from build123d import *

# Parameters (mm, degrees)
F0_W        = 85
F0_H        = 85
F1_DEPTH    = 3
F2_R        = 5
F3_DEPTH    = 7
F4_R        = 8
F5_R        = 2
F6_T1_DEPTH = 7


# Not quite as in the source:
# - a fillet or chamfer that OpenCascade refuses, or shapes differently, is made with other operations: its cross-section is extruded or revolved along the edge and cut away or added


with BuildPart() as f1:
    # F0 (on Top) → F1 (new body)
    with BuildSketch(Plane.XY):
        Rectangle(F0_W, F0_H)
        Polygon((-37.5, -6), (-37.5, 6), (-37.5, 37.5), (37.5, 37.5), (37.5, 6), (37.5, -6), (37.5, -37.5), (-37.5, -37.5), align=None, mode=Mode.SUBTRACT)
        Polygon((-35.1, -35.1), (-35.1, -5.85), (-36, -6), (-37.5, -6), (-37.5, -37.5), (37.5, -37.5), (37.5, -6), (36, -6), (35.1, -5.85), (35.1, -35.1), align=None)
        Polygon((-36, 6), (-35.1, 5.85), (-35.1, 35.1), (35.1, 35.1), (35.1, 5.85), (36, 6), (37.5, 6), (37.5, 37.5), (-37.5, 37.5), (-37.5, 6), align=None)
        Polygon((-32, 5.3333333333), (-32, 33), (32, 33), (32, 5.3333333333), (35.1, 5.85), (35.1, 35.1), (-35.1, 35.1), (-35.1, 5.85), align=None)
        with BuildLine():
            Line((-32, 4.582575695), (-32, 5.3333333333))
            Line((-32, 5.3333333333), (-35.1, 5.85))
            Line((-35.1, 5.85), (-35.1, -5.85))
            Line((-35.1, -5.85), (-32, -5.3333333333))
            Line((-32, -5.3333333333), (-32, -4.582575695))
            ThreePointArc((-32, -4.582575695), (-35, 0), (-32, 4.582575695))
        make_face()
        Polygon((-35.1, -5.85), (-35.1, 5.85), (-36, 6), (-36, -6), align=None)
        with BuildLine():
            ThreePointArc((-30, 5), (-31.0215482184, 4.8945315647), (-32, 4.582575695))
            Line((-32, 4.582575695), (-32, 2.2360679775))
            ThreePointArc((-32, 2.2360679775), (-28.7752551286, 2.7386127875), (-27, 0))
            ThreePointArc((-27, 0), (-28.7752551286, -2.7386127875), (-32, -2.2360679775))
            Line((-32, -2.2360679775), (-32, -4.582575695))
            ThreePointArc((-32, -4.582575695), (-31.0215482184, -4.8945315647), (-30, -5))
            ThreePointArc((-30, -5), (-26.4644660941, -3.5355339059), (-25, 0))
            ThreePointArc((-25, 0), (-26.4644660941, 3.5355339059), (-30, 5))
        make_face()
        with BuildLine():
            Line((-30, 5), (-32, 5.3333333333))
            Line((-32, 5.3333333333), (-32, 4.582575695))
            ThreePointArc((-32, 4.582575695), (-31.0215482184, 4.8945315647), (-30, 5))
        make_face()
        with BuildLine():
            ThreePointArc((-30, -5), (-31.0215482184, -4.8945315647), (-32, -4.582575695))
            Line((-32, -4.582575695), (-32, -5.3333333333))
            Line((-32, -5.3333333333), (-30, -5))
        make_face()
        Polygon((-32, -5.3333333333), (-35.1, -5.85), (-35.1, -35.1), (35.1, -35.1), (35.1, -5.85), (32, -5.3333333333), (32, -33), (-32, -33), align=None)
        with BuildLine():
            Line((35.1, 5.85), (32, 5.3333333333))
            Line((32, 5.3333333333), (32, 4.582575695))
            ThreePointArc((32, 4.582575695), (34.1833001327, 2.7386127875), (35, 0))
            ThreePointArc((35, 0), (34.1833001327, -2.7386127875), (32, -4.582575695))
            Line((32, -4.582575695), (32, -5.3333333333))
            Line((32, -5.3333333333), (35.1, -5.85))
            Line((35.1, -5.85), (35.1, 5.85))
        make_face()
        with BuildLine():
            Line((32, 4.582575695), (32, 5.3333333333))
            Line((32, 5.3333333333), (30, 5))
            ThreePointArc((30, 5), (31.0215482184, 4.8945315647), (32, 4.582575695))
        make_face()
        with BuildLine():
            ThreePointArc((32, -4.582575695), (31.0215482184, -4.8945315647), (30, -5))
            Line((30, -5), (32, -5.3333333333))
            Line((32, -5.3333333333), (32, -4.582575695))
        make_face()
        with BuildLine():
            Line((32, 2.2360679775), (32, 4.582575695))
            ThreePointArc((32, 4.582575695), (31.0215482184, 4.8945315647), (30, 5))
            ThreePointArc((30, 5), (25, 0), (30, -5))
            ThreePointArc((30, -5), (31.0215482184, -4.8945315647), (32, -4.582575695))
            Line((32, -4.582575695), (32, -2.2360679775))
            ThreePointArc((32, -2.2360679775), (27, 0), (32, 2.2360679775))
        make_face()
        with BuildLine():
            ThreePointArc((35, 0), (34.1833001327, 2.7386127875), (32, 4.582575695))
            Line((32, 4.582575695), (32, 2.2360679775))
            ThreePointArc((32, 2.2360679775), (32.7386127875, 1.2247448714), (33, 0))
            ThreePointArc((33, 0), (32.7386127875, -1.2247448714), (32, -2.2360679775))
            Line((32, -2.2360679775), (32, -4.582575695))
            ThreePointArc((32, -4.582575695), (34.1833001327, -2.7386127875), (35, 0))
        make_face()
        with BuildLine():
            Line((-32, 2.2360679775), (-32, 4.582575695))
            ThreePointArc((-32, 4.582575695), (-35, 0), (-32, -4.582575695))
            Line((-32, -4.582575695), (-32, -2.2360679775))
            ThreePointArc((-32, -2.2360679775), (-33, 0), (-32, 2.2360679775))
        make_face()
        Polygon((36, 6), (35.1, 5.85), (35.1, -5.85), (36, -6), align=None)
    extrude(amount=F1_DEPTH)

    # F2
    f2_edges = [f1.edges().sort_by_distance(p)[0] for p in [
        (-42.5, 42.5, 1.5),
        (-42.5, -42.5, 1.5),
        (42.5, -42.5, 1.5),
        (42.5, 42.5, 1.5),
    ]]
    fillet(f2_edges, radius=F2_R)

    # F0 (on Top) → F3 (join)
    with BuildSketch(Plane.XY):
        with BuildLine():
            Line((-32, 4.582575695), (-32, 5.3333333333))
            Line((-32, 5.3333333333), (-35.1, 5.85))
            Line((-35.1, 5.85), (-35.1, -5.85))
            Line((-35.1, -5.85), (-32, -5.3333333333))
            Line((-32, -5.3333333333), (-32, -4.582575695))
            ThreePointArc((-32, -4.582575695), (-35, 0), (-32, 4.582575695))
        make_face()
        with BuildLine():
            Line((-30, 5), (-32, 5.3333333333))
            Line((-32, 5.3333333333), (-32, 4.582575695))
            ThreePointArc((-32, 4.582575695), (-31.0215482184, 4.8945315647), (-30, 5))
        make_face()
        with BuildLine():
            ThreePointArc((-30, 5), (-31.0215482184, 4.8945315647), (-32, 4.582575695))
            Line((-32, 4.582575695), (-32, 2.2360679775))
            ThreePointArc((-32, 2.2360679775), (-28.7752551286, 2.7386127875), (-27, 0))
            ThreePointArc((-27, 0), (-28.7752551286, -2.7386127875), (-32, -2.2360679775))
            Line((-32, -2.2360679775), (-32, -4.582575695))
            ThreePointArc((-32, -4.582575695), (-31.0215482184, -4.8945315647), (-30, -5))
            ThreePointArc((-30, -5), (-26.4644660941, -3.5355339059), (-25, 0))
            ThreePointArc((-25, 0), (-26.4644660941, 3.5355339059), (-30, 5))
        make_face()
        with BuildLine():
            Line((-32, 2.2360679775), (-32, 4.582575695))
            ThreePointArc((-32, 4.582575695), (-35, 0), (-32, -4.582575695))
            Line((-32, -4.582575695), (-32, -2.2360679775))
            ThreePointArc((-32, -2.2360679775), (-33, 0), (-32, 2.2360679775))
        make_face()
        with BuildLine():
            ThreePointArc((-30, -5), (-31.0215482184, -4.8945315647), (-32, -4.582575695))
            Line((-32, -4.582575695), (-32, -5.3333333333))
            Line((-32, -5.3333333333), (-30, -5))
        make_face()
        Polygon((-32, -5.3333333333), (-35.1, -5.85), (-35.1, -35.1), (35.1, -35.1), (35.1, -5.85), (32, -5.3333333333), (32, -33), (-32, -33), align=None)
        Polygon((-35.1, -35.1), (-35.1, -5.85), (-36, -6), (-37.5, -6), (-37.5, -37.5), (37.5, -37.5), (37.5, -6), (36, -6), (35.1, -5.85), (35.1, -35.1), align=None)
        Polygon((-36, 6), (-35.1, 5.85), (-35.1, 35.1), (35.1, 35.1), (35.1, 5.85), (36, 6), (37.5, 6), (37.5, 37.5), (-37.5, 37.5), (-37.5, 6), align=None)
        Polygon((-32, 5.3333333333), (-32, 33), (32, 33), (32, 5.3333333333), (35.1, 5.85), (35.1, 35.1), (-35.1, 35.1), (-35.1, 5.85), align=None)
        with BuildLine():
            ThreePointArc((32, -4.582575695), (31.0215482184, -4.8945315647), (30, -5))
            Line((30, -5), (32, -5.3333333333))
            Line((32, -5.3333333333), (32, -4.582575695))
        make_face()
        with BuildLine():
            Line((32, 2.2360679775), (32, 4.582575695))
            ThreePointArc((32, 4.582575695), (31.0215482184, 4.8945315647), (30, 5))
            ThreePointArc((30, 5), (25, 0), (30, -5))
            ThreePointArc((30, -5), (31.0215482184, -4.8945315647), (32, -4.582575695))
            Line((32, -4.582575695), (32, -2.2360679775))
            ThreePointArc((32, -2.2360679775), (27, 0), (32, 2.2360679775))
        make_face()
        with BuildLine():
            Line((32, 4.582575695), (32, 5.3333333333))
            Line((32, 5.3333333333), (30, 5))
            ThreePointArc((30, 5), (31.0215482184, 4.8945315647), (32, 4.582575695))
        make_face()
        with BuildLine():
            ThreePointArc((35, 0), (34.1833001327, 2.7386127875), (32, 4.582575695))
            Line((32, 4.582575695), (32, 2.2360679775))
            ThreePointArc((32, 2.2360679775), (32.7386127875, 1.2247448714), (33, 0))
            ThreePointArc((33, 0), (32.7386127875, -1.2247448714), (32, -2.2360679775))
            Line((32, -2.2360679775), (32, -4.582575695))
            ThreePointArc((32, -4.582575695), (34.1833001327, -2.7386127875), (35, 0))
        make_face()
        with BuildLine():
            Line((35.1, 5.85), (32, 5.3333333333))
            Line((32, 5.3333333333), (32, 4.582575695))
            ThreePointArc((32, 4.582575695), (34.1833001327, 2.7386127875), (35, 0))
            ThreePointArc((35, 0), (34.1833001327, -2.7386127875), (32, -4.582575695))
            Line((32, -4.582575695), (32, -5.3333333333))
            Line((32, -5.3333333333), (35.1, -5.85))
            Line((35.1, -5.85), (35.1, 5.85))
        make_face()
    extrude(amount=F3_DEPTH)

    # F4
    f4_edges = [f1.edges().sort_by_distance(p)[0] for p in [
        (-37.5, -37.5, 5),
        (37.5, -37.5, 5),
        (37.5, 37.5, 5),
        (-37.5, 37.5, 5),
    ]]
    fillet(f4_edges, radius=F4_R)

    # F5
    f5_edges = [f1.edges().sort_by_distance(p)[0] for p in [
        (32, -33, 3.5),
        (-32, -33, 3.5),
        (-32, 33, 3.5),
        (32, 33, 3.5),
    ]]
    fillet(f5_edges, radius=F5_R)

    # F6: fillet of radius 5 on 4 edges, made by hand

    # F6_s2 → F6_t1 (join)
    with BuildSketch(Plane.XY):
        with BuildLine():
            ThreePointArc((30, -5), (31.472135955, -6.7639320225), (32, -9))
            Line((32, -9), (32, -5.3333333333))
            Line((32, -5.3333333333), (30, -5))
        make_face()
        with BuildLine():
            ThreePointArc((32, 9), (31.472135955, 6.7639320225), (30, 5))
            Line((30, 5), (32, 5.3333333333))
            Line((32, 5.3333333333), (32, 9))
        make_face()
        with BuildLine():
            ThreePointArc((-32, 9), (-31.472135955, 6.7639320225), (-30, 5))
            Line((-30, 5), (-32, 5.3333333333))
            Line((-32, 5.3333333333), (-32, 9))
        make_face()
        with BuildLine():
            ThreePointArc((-30, -5), (-31.472135955, -6.7639320225), (-32, -9))
            Line((-32, -9), (-32, -5.3333333333))
            Line((-32, -5.3333333333), (-30, -5))
        make_face()
    extrude(amount=F6_T1_DEPTH)


solid = f1.part
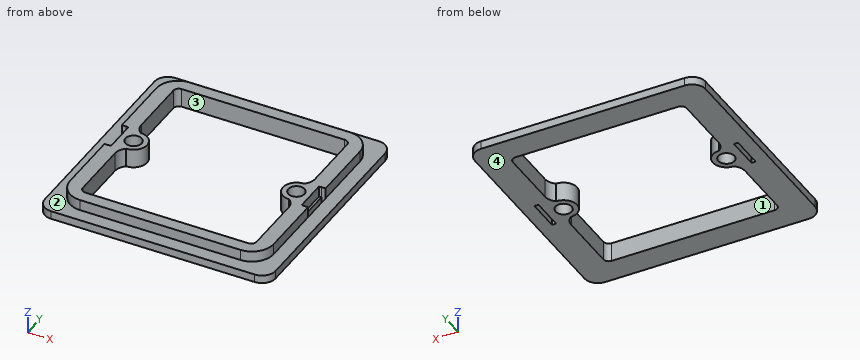
Part model, mm, in its own coordinate system. Face numbers are marked on the shaded views. A direction names the side the tool comes from. Round coordinates to 2 decimals unless told otherwise and drop trailing zeros. Write each loop counter-clockwise with the first axis right and the second up, starting at its lowest first coordinate (ties: lowest second). Pieces come first, ordered by that corner, then holes. Notation, with made-up numbers: (89.5, 75) - (125.5, 75) arc R25 cw to (125.5, 94) - close; hole circle Ø8 at (29.25, 55). An arc over 180 degrees is marked (long way). Use CSV: the item, a comma, the result in double quotes.
Item 1: Pull direction Y, two halves, no side cores. Call the marked faces 3 and 4: pulls with the +Y half, pulls with the -Y half, needs draft (parallel to the pull), parting line crosses it, or undercut.
Results list:
face 3,"undercut"
face 4,"needs draft"
Item 2: Slice it at B-B, the plane y = 28. Write the cut outline in (x, z).
Results list:
outline,"(-42.5, 0) - (-32, 0) - (-32, 7) - (-37.5, 7) - (-37.5, 3) - (-42.5, 3) - close; (32, 0) - (42.5, 0) - (42.5, 3) - (37.5, 3) - (37.5, 7) - (32, 7) - close"
Item 3: Wall check: L1, parallel to Y at x = -30, z = 2.75; L2, parallel to Y at x = -30, z = 5.25; L3, parallel to Y at x = 19.5, z = 4. Give the ranges that are in metal, low to high.
Results list:
L1,"y = -42.5 to -33, -5 to -3, 3 to 5, 33 to 42.5"
L2,"y = -37.48 to -33, -5 to -3, 3 to 5, 33 to 37.48"
L3,"y = -37.5 to -33, 33 to 37.5"
Item 4: Slice it at A-A, the plane x = -6.5. Write the cut outline in (y, z).
Results list:
outline,"(-42.5, 0) - (-33, 0) - (-33, 7) - (-37.5, 7) - (-37.5, 3) - (-42.5, 3) - close; (33, 0) - (42.5, 0) - (42.5, 3) - (37.5, 3) - (37.5, 7) - (33, 7) - close"
Item 5: Tool access for the marked faces 1 and 2: list every direction of +Z, -Z, +X, -X, +Y, -Y with a clear straight run to the whole face (end or side of a thin tool).
Results list:
face 1,"+Z, -Z"
face 2,"+Z"
Item 6: Slice it at C-C, the plane y = 0. Write the cut outline in (x, z), then the cut area to 3 significant figures.
Results list:
outline,"(-42.5, 0) - (-37.5, 0) - (-37.5, 3) - (-42.5, 3) - close; (-36, 0) - (-33, 0) - (-33, 7) - (-35.1, 7) - (-35.1, 3) - (-36, 3) - close; (-27, 0) - (-25, 0) - (-25, 7) - (-27, 7) - close; (25, 0) - (27, 0) - (27, 7) - (25, 7) - close; (33, 0) - (36, 0) - (36, 3) - (35.1, 3) - (35.1, 7) - (33, 7) - close; (37.5, 0) - (42.5, 0) - (42.5, 3) - (37.5, 3) - close"
area,"92.8 mm²"
Item 7: Flat gauge pins, fed straight in: P1, Ø1.5, axis at x = -18.5, z = 4.5, coming from the +Y side; P2, Ø1.6, axis at x = -36.5, z = 5, coming from the +Y side; P3, Ø1.2, axis at y = 12.5, z = 4, coming from the -X side. Where does each tip first touch, or does it go through?
Results list:
P1,"stops at y = 37.5"
P2,"stops at y = 34.56"
P3,"stops at x = -37.5"
Item 8: Slice it at D-D, the plane z = 1.5. Count the separate pieces of the cut face and the enclosed holes in it, then the cut area to 3 significant figures.
Results list:
separate pieces,"1"
enclosed holes,"5"
area,"3,020 mm²"
